Here's how the part is built. I have some questions about the finished solid (model axes, mm). Face numbers are marked on the shaded views. A direction names the side the tool comes from. Give positions to 0.01 mm unless a question says otherwise; leave off trailing zeros. Write each loop counter-clockwise with the first axis right and the second up, starting at its lowest first coordinate (ties: lowest second). Pieces come first, ordered by that corner, then holes. Notation, with made-up numbers: (9, 66.25) - (32, 66.25) arc R36 cw to (32, 100.25) - close; hole circle Ø4 at (62.25, -19). An arc over 180 degrees is marked (long way). Use a Markdown table: item, result.
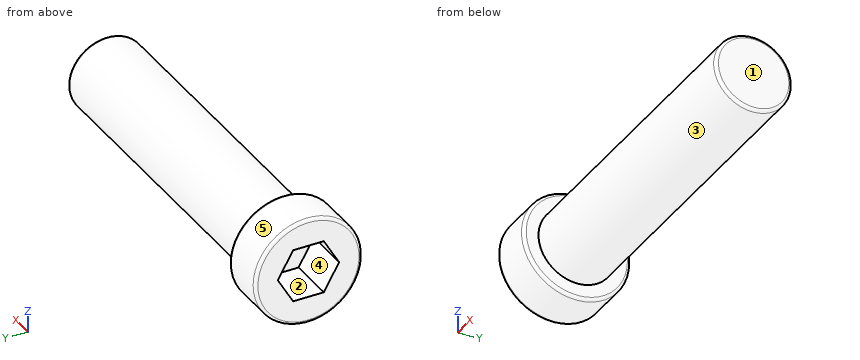
```python
from build123d import *

# Parameters (mm, degrees)
FILLET1_R          = 0.2
CUT_EXTRUDE1_DEPTH = 3


with BuildPart() as part:
    # Sketch1 → Revolve1 (revolve)
    with BuildSketch(Plane.XY):
        Polygon((0, 0), (-24, 0), (-24, 3.5), (-21, 3.5), (-21, 2.5), (0, 2.5), align=None)
    revolve(axis=Axis((0, 0, 0), (-1, 0, 0)))

    # Fillet1
    fillet1_edges = [part.edges().sort_by_distance(p)[0] for p in [
        (0, -2.5, 0),
        (-21, -3.5, 0),
        (-24, -3.5, 0),
    ]]
    fillet(fillet1_edges, radius=FILLET1_R)

    # Sketch2 → Cut-Extrude1 (cut)
    with BuildSketch(Plane.ZY.offset(24)):
        Polygon((0, 2), (-1.732050808, 1), (-1.732050808, -1), (0, -2), (1.732050808, -1), (1.732050808, 1), align=None)
    extrude(amount=-CUT_EXTRUDE1_DEPTH, mode=Mode.SUBTRACT)


solid = part.part
```
Item 1: For the marked faces 4 and 5, which set-ups out of +Z, -Z, +X, -X, +Y, -Y let a thin tool reach every point of the face, with its end or its side?
Values:
| item | result |
|---|---|
| face 4 | -X |
| face 5 | +X, -X |
Item 2: Will these pins go through, and if not, where does the flat tip stop? pin 1 Ø1 at (x, z) = (-16, 0) entering from +Y; pin 2 Ø3 at (x, y) = (-7, -2) entering from -Z.
Values:
| item | result |
|---|---|
| pin 1 | stops at y = 2.5 |
| pin 2 | stops at z = -2.45 |
Item 3: I need wall thicknesses on line 1 along X through (y, z) = (1, -3); line 2 along Y through (x, z) = (-7, 1.5); line 3 along Z through (x, y) = (-15.5, 0). Which ranges of each line are inside material? Lowest first, please. Write a range as [from, to].
Values:
| item | result |
|---|---|
| line 1 | x = [-24, -21] |
| line 2 | y = [-2, 2] |
| line 3 | z = [-2.5, 2.5] |
Item 4: If we section it at A-A, the plane y = 0: Write out the boundary of the cut face in (x, z), plus the area to 3 significant figures.
Values:
| item | result |
|---|---|
| outline | (-24, -3.3) arc R0.2 ccw to (-23.8, -3.5) - (-21.2, -3.5) arc R0.2 ccw to (-21, -3.3) - (-21, -2.5) - (-0.2, -2.5) arc R0.2 ccw to (0, -2.3) - (0, 2.3) arc R0.2 ccw to (-0.2, 2.5) - (-21, 2.5) - (-21, 3.3) arc R0.2 ccw to (-21.2, 3.5) - (-23.8, 3.5) arc R0.2 ccw to (-24, 3.3) - (-24, 1.73) - (-21, 1.73) - (-21, -1.73) - (-24, -1.73) - close |
| area | 116 mm2 |
Item 5: If we section it at B-B, the plane x = -15: Write out the boundary of the cut face in (y, z), plus the area to 3 significant figures.
Values:
| item | result |
|---|---|
| outline | circle Ø5 at (0, 0) |
| area | 19.6 mm2 |
Item 6: Thinking about a two-plate mould opening in Y: for the marked faces 1, 2 and 3, which applies, +Y half, -Y half, draft (parallel to the pull), parting line (faces both ways), or undercut?
Values:
| item | result |
|---|---|
| face 1 | draft |
| face 2 | undercut |
| face 3 | parting line |
